from build123d import *

# Parameters (mm, degrees)
SKETCH_1_W     = 1
SKETCH_1_H     = 6
CHAMFER_1_SIZE = 0.1


with BuildPart() as part:
    # 草图1 → 旋转1 (revolve)
    with BuildSketch(Plane.XY, mode=Mode.PRIVATE) as revolve_1_sk:
        with Locations((-0.5, 4.5)):
            Rectangle(SKETCH_1_W, SKETCH_1_H)
    revolve(revolve_1_sk.sketch.rotate(Axis((-11.624698891, 0, 0), (1, 0, 0)), 90), axis=Axis((-11.624698891, 0, 0), (1, 0, 0)))

    # 倒角1
    chamfer_1_edges = [part.edges().sort_by_distance(p)[0] for p in [
        (-1, 0, -1.5),
        (-1, 0, -7.5),
        (0, 0, -7.5),
        (0, 0, -1.5),
    ]]
    chamfer(chamfer_1_edges, length=CHAMFER_1_SIZE)


solid = part.part
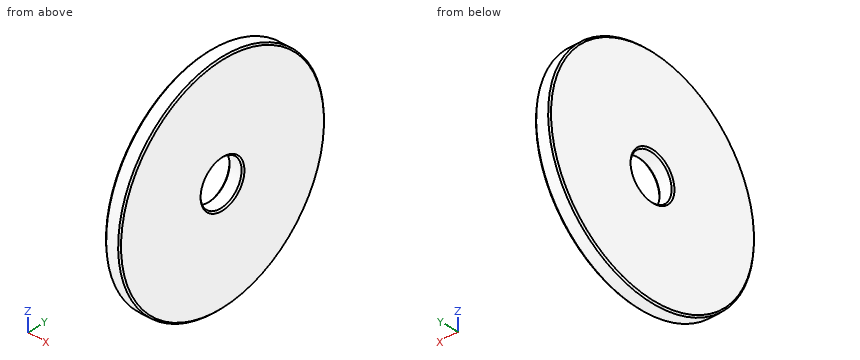
Geometry: final body of the model. Coordinates: model frame, mm. Give positions to 0.01 mm unless a question says otherwise; leave off trailing zeros. Loops run counter-clockwise (first coordinate to the right, second up) from the corner with the lowest first, then second, coordinate; pieces in that order, holes last. Notation, with made-up numbers: (-3, -9) -> (51, -9) arc R21 cw to (51, 16) -> close; hole circle Ø1 at (33.5, 67). An arc over 180 degrees is marked (long way). Put each result on its own line as item: value.
1. Cut plane C-C (x = -0.6). Return the cut outline in (y, z).
Taken from the geometry:
outline: circle Ø15 at (0, 0); hole circle Ø3 at (0, 0)
2. Cut plane A-A (y = 0). Return the cut outline in (x, z).
Taken from the geometry:
outline: (-1, -7.4) -> (-0.9, -7.5) -> (-0.1, -7.5) -> (0, -7.4) -> (0, -1.6) -> (-0.1, -1.5) -> (-0.9, -1.5) -> (-1, -1.6) -> close; (-1, 1.6) -> (-0.9, 1.5) -> (-0.1, 1.5) -> (0, 1.6) -> (0, 7.4) -> (-0.1, 7.5) -> (-0.9, 7.5) -> (-1, 7.4) -> close
3. Ray query, line 1 along Y through (x, z) = (-0.35, 0); line 2 along Z through (x, y) = (-0.4, -1.25); line 3 along Z through (x, y) = (-0.25, -4.5). Return the intervals inside material, ascending. Write a range as [from, to].
Taken from the geometry:
line 1: y = [-7.5, -1.5], [1.5, 7.5]
line 2: z = [-7.4, -0.83], [0.83, 7.4]
line 3: z = [-6, 6]
